Build history of the part. All positions in model axes, mm. A direction names the side the tool comes from. Give positions to 0.01 mm unless a question says otherwise; leave off trailing zeros. Write each loop counter-clockwise with the first axis right and the second up, starting at its lowest first coordinate (ties: lowest second). Pieces come first, ordered by that corner, then holes. Notation, with made-up numbers: (30.25, 16) -> (57.25, 16) arc R26 ccw to (57.25, 41) -> close; hole circle Ø3 at (61, 34.5). An arc over 180 degrees is marked (long way). One line per question, with ' | ' between items. Start each with the question number.
(1) Tool access for faces 4 (the flat face through (0, 13, 0.75)), 5 (the flat face through (0, 0, 0)): list every direction of +Z, -Z, +X, -X, +Y, -Y with a clear straight run to the whole face (end or side of a thin tool).
(2) Band-saw the part on A-A, the plane y = 7. Give the cut face in (x, z), and give its area (3 significant figures).
(3) Pin check, flat tips, straight feed: P1, Ø1, axis at x = 1, z = -1, coming from the +Y side; P2, Ø1.7, axis at x = 0, z = 0.5, coming from the -Y side. Stop position of each tip, or through.
(4) Drill centre lines: probe 1 along Y at (x, z) = (0.9, 0.25); probe 2 along X at (y, z) = (12, 0.9); probe 3 along Y at (x, z) = (-1, 0.6). Where is each one in solid material? Low to high. Write a range as from..to.
(5) Pull direction X, two halves, no side cores. Call faces 1 (the flat face through (1, 11.85, -1)), 2 (the flat face through (0, 13, -0.75)), 3 (the cylindrical face through (-0.24, 6.006, 0.763)): released by +X, released by -X, zero draft, split by the parting line, or undercut.
from build123d import *

# Parameters (mm, degrees)
CUT_EXTRUDE2_DEPTH = 13.123312284


with BuildPart() as part:
    # Sketch1 → Revolve1 (revolve)
    with BuildSketch(Plane(origin=(0, 0, 0), x_dir=(0, 0, -1), z_dir=(1, 0, 0)), mode=Mode.PRIVATE) as revolve1_sk:
        with BuildLine():
            ThreePointArc((0.8, 11.7), (0.843933983, 11.806066017), (0.95, 11.85))
            Line((0.95, 11.85), (1.66, 11.85))
            ThreePointArc((1.66, 11.85), (1.766066017, 11.893933983), (1.81, 12))
            Line((1.81, 12), (1.81, 12.728765944))
            ThreePointArc((1.81, 12.728765944), (1.783686321, 12.840410154), (1.710284562, 12.928552205))
            ThreePointArc((1.710284562, 12.928552205), (1.354338624, 13.156968158), (0.968464524, 13.330093943))
            ThreePointArc((0.968464524, 13.330093943), (0.922426778, 13.343109085), (0.875, 13.349399447))
            Line((0.875, 13.349399447), (0.875, 12.256185485))
            ThreePointArc((0.875, 12.256185485), (0.845317103, 12.166609847), (0.768016069, 12.112485736))
            ThreePointArc((0.768016069, 12.112485736), (0.646674627, 12.079247272), (0.523906049, 12.051744226))
            ThreePointArc((0.523906049, 12.051744226), (0.263227569, 12.012967451), (0, 12))
            Line((0, 12), (0, 0))
            Line((0, 0), (0.65, 0))
            Line((0.65, 0), (0.8, 0.15))
            Line((0.8, 0.15), (0.8, 11.7))
        make_face()
    revolve(revolve1_sk.sketch.rotate(Axis((0, 13.5, 0), (0, -1, 0)), 180), axis=Axis((0, 13.5, 0), (0, -1, 0)))


with BuildPart() as body_2:
    # Sketch1_3 → Revolve2 (revolve)
    with BuildSketch(Plane(origin=(0, 0, 0), x_dir=(0, 0, -1), z_dir=(1, 0, 0)), mode=Mode.PRIVATE) as revolve2_sk:
        with BuildLine():
            Line((0.875, 12.256185485), (0.875, 13.349399447))
            ThreePointArc((0.875, 13.349399447), (0.865004507, 13.349849828), (0.855, 13.35))
            Line((0.855, 13.35), (0.725, 13.22))
            Line((0.725, 13.22), (0.725, 12.29691396))
            ThreePointArc((0.725, 12.29691396), (0.668295774, 12.138368245), (0.523906049, 12.051744226))
            ThreePointArc((0.523906049, 12.051744226), (0.646674627, 12.079247272), (0.768016069, 12.112485736))
            ThreePointArc((0.768016069, 12.112485736), (0.845317103, 12.166609847), (0.875, 12.256185485))
        make_face()
    revolve(revolve2_sk.sketch.rotate(Axis((0, 13.5, 0), (0, -1, 0)), 180), axis=Axis((0, 13.5, 0), (0, -1, 0)))

    # Sketch2 → Cut-Extrude2 (cut, through all)
    with BuildSketch(Plane.XZ.offset(-11.85)):
        Polygon((-0.433012702, 0.75), (-0.866025404, 0), (-0.433012702, -0.75), (0.433012702, -0.75), (0.866025404, 0), (0.433012702, 0.75), align=None)
    extrude(amount=-CUT_EXTRUDE2_DEPTH, mode=Mode.SUBTRACT)


with BuildPart() as part_1:
    add(part.part)

    # Combine1: union body 2
    add(body_2.part)


solid = part_1.part
Results:
1) face 4: +Y | face 5: +Z, -Z, +X, -X, -Y
2) outline: circle Ø1.6 at (0, 0) | area: 2.01 mm²
3) P1: stops at y = 13.34 | P2: stops at y = 0
4) probe 1: y = 11.85..13.34 | probe 2: x = -1.57..1.57 | probe 3: y = 11.85..13.25
5) face 1: zero draft | face 2: undercut | face 3: split by the parting line
